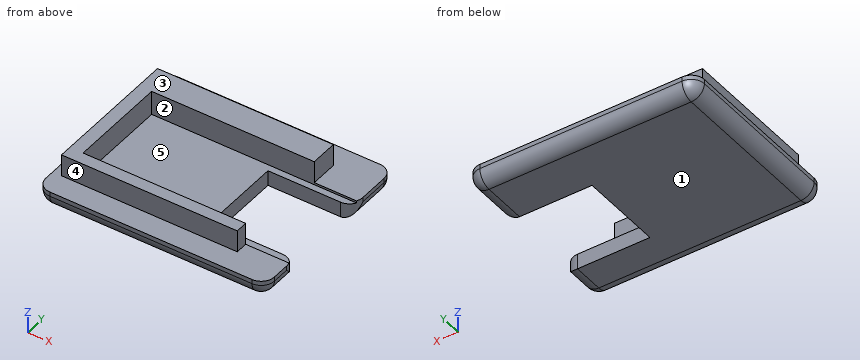
from build123d import *

# Parameters (mm, degrees)
SKETCH1_W           = 52
SKETCH1_H           = 42
BOSS_EXTRUDE1_DEPTH = 4
SKETCH2_W           = 40
SKETCH2_H           = 31.5
BOSS_EXTRUDE2_DEPTH = 5
SKETCH4_W           = 50
SKETCH4_H           = 22.5
CUT_EXTRUDE2_DEPTH  = 5.5
SKETCH5_W           = 19.5
SKETCH5_H           = 19
CUT_EXTRUDE3_DEPTH  = 10
FILLET2_R           = 3


with BuildPart() as part:
    # Sketch1 → Boss-Extrude1 (new body)
    with BuildSketch(Plane.XY):
        Rectangle(SKETCH1_W, SKETCH1_H)
    extrude(amount=BOSS_EXTRUDE1_DEPTH)

    # Sketch2 → Boss-Extrude2 (add)
    with BuildSketch(Plane.XY.offset(4)):
        with Locations((-4, 0)):
            Rectangle(SKETCH2_W, SKETCH2_H)
    extrude(amount=BOSS_EXTRUDE2_DEPTH)

    # Sketch4 → Cut-Extrude2 (cut)
    with BuildSketch(Plane.XY.offset(9)):
        with Locations((4, -1.75)):
            Rectangle(SKETCH4_W, SKETCH4_H)
    extrude(amount=-CUT_EXTRUDE2_DEPTH, mode=Mode.SUBTRACT)

    # Sketch5 → Cut-Extrude3 (cut)
    with BuildSketch(Plane.XY.offset(3.5)):
        with Locations((16.25, -1.5)):
            Rectangle(SKETCH5_W, SKETCH5_H)
    extrude(amount=-CUT_EXTRUDE3_DEPTH, mode=Mode.SUBTRACT)

    # Fillet2
    fillet2_edges = [part.edges().sort_by_distance(p)[0] for p in [
        (26, -16, 0),
        (26, 14.5, 0),
        (26, 8, 1.75),
        (26, -11, 1.75),
        (26, -21, 2),
        (-26, -21, 2),
        (0, -21, 0),
        (-26, 0, 0),
        (0, 21, 0),
        (-26, 21, 2),
        (26, 21, 2),
    ]]
    fillet(fillet2_edges, radius=FILLET2_R)


solid = part.part
Work out the finished part from the listing and answer in its coordinate system (mm). Face numbers are marked on the shaded views. A direction names the side the tool comes from. Give positions to 0.01 mm unless a question says otherwise; leave off trailing zeros. Loops run counter-clockwise (first coordinate to the right, second up) from the corner with the lowest first, then second, coordinate; pieces in that order, holes last. Notation, with made-up numbers: (25.25, 61) - (82.25, 61) arc R22 ccw to (82.25, 86) - close; hole circle Ø2 at (-14, 54.5). An arc over 180 degrees is marked (long way). Answer in a Markdown table with one row per item.
(1) Consider L1, parallel to Y at x = -17.5, z = 8.25; L2, parallel to X at y = -15.5, z = 8.5; L3, parallel to X at y = -6.5, z = 3. Determine where each line is inside the solid, lowest interval first. Write a range as [from, to].
Results list:
| item | result |
|---|---|
| L1 | y = [-15.75, -13], [9.5, 15.75] |
| L2 | x = [-24, 16] |
| L3 | x = [-26, 6.5] |
(2) A tool of negligible diameter and unlimited length cuts with its end or side. For the marked faces 1 and 2, from which of +Z, -Z, +X, -X, +Y, -Y can it reach the whole face along a straight path? Write none if from no direction.
Results list:
| item | result |
|---|---|
| face 1 | -Z, +X, -X, +Y, -Y |
| face 2 | +Z, +X |
(3) Section A-A (x = 18.5) is taken. Give the vertices of the cut face in (y, z), and give its area (3 significant figures).
Results list:
| item | result |
|---|---|
| outline | (-21, 3) arc R3 ccw to (-18, 0) - (-11, 0) - (-11, 3.5) - (-13, 3.5) - (-13, 4) - (-21, 4) - close; (8, 0) - (18, 0) arc R3 ccw to (21, 3) - (21, 4) - (9.5, 4) - (9.5, 3.5) - (8, 3.5) - close |
| area | 86.4 mm² |
(4) Flat-ended cylindrical pins translate along their axes: pin 1 Ø3 at (y, z) = (0, 2) entering from +X; pin 2 Ø2.5 at (x, z) = (-4, 6.5) entering from -Y; pin 3 Ø3 at (y, z) = (-2.5, 6.5) entering from +X. Find the tip coordinate at first contact, or state that the pin passes through.
Results list:
| item | result |
|---|---|
| pin 1 | stops at x = 6.5 |
| pin 2 | stops at y = -15.75 |
| pin 3 | stops at x = -21 |
(5) Section D-D (z = 1.75) is taken. Give the vertices of the cut face in (x, y), and give its area (3 significant figures).
Results list:
| item | result |
|---|---|
| outline | (-25.73, -18) arc R2.73 ccw to (-23, -20.73) - (23, -20.73) arc R2.73 ccw to (25.73, -18) - (25.73, -12.75) arc R3 ccw to (23, -11) - (6.5, -11) - (6.5, 8) - (23, 8) arc R3 ccw to (25.73, 9.75) - (25.73, 18) arc R2.73 ccw to (23, 20.73) - (-23, 20.73) arc R2.73 ccw to (-25.73, 18) - close |
| area | 1,760 mm² |
(6) Section C-C (x = -10.5) is taken. Give the vertices of the cut face in (y, z).
Results list:
| item | result |
|---|---|
| outline | (-21, 3) arc R3 ccw to (-18, 0) - (18, 0) arc R3 ccw to (21, 3) - (21, 4) - (15.75, 4) - (15.75, 9) - (9.5, 9) - (9.5, 3.5) - (-13, 3.5) - (-13, 9) - (-15.75, 9) - (-15.75, 4) - (-21, 4) - close |
(7) For a pull along Y with two mould halves and no side action, classify the marked faces 3, 4 and 5 as pulls with the +Y half, pulls with the -Y half, needs draft (parallel to the pull), parting line crosses it, or undercut.
Results list:
| item | result |
|---|---|
| face 3 | needs draft |
| face 4 | pulls with the -Y half |
| face 5 | undercut |
(8) Section B-B (z = 7.5) is taken. Give the vertices of the cut face in (x, y), and give its area (4 significant figures).
Results list:
| item | result |
|---|---|
| outline | (-24, -15.75) - (16, -15.75) - (16, -13) - (-21, -13) - (-21, 9.5) - (16, 9.5) - (16, 15.75) - (-24, 15.75) - close |
| area | 427.5 mm² |
